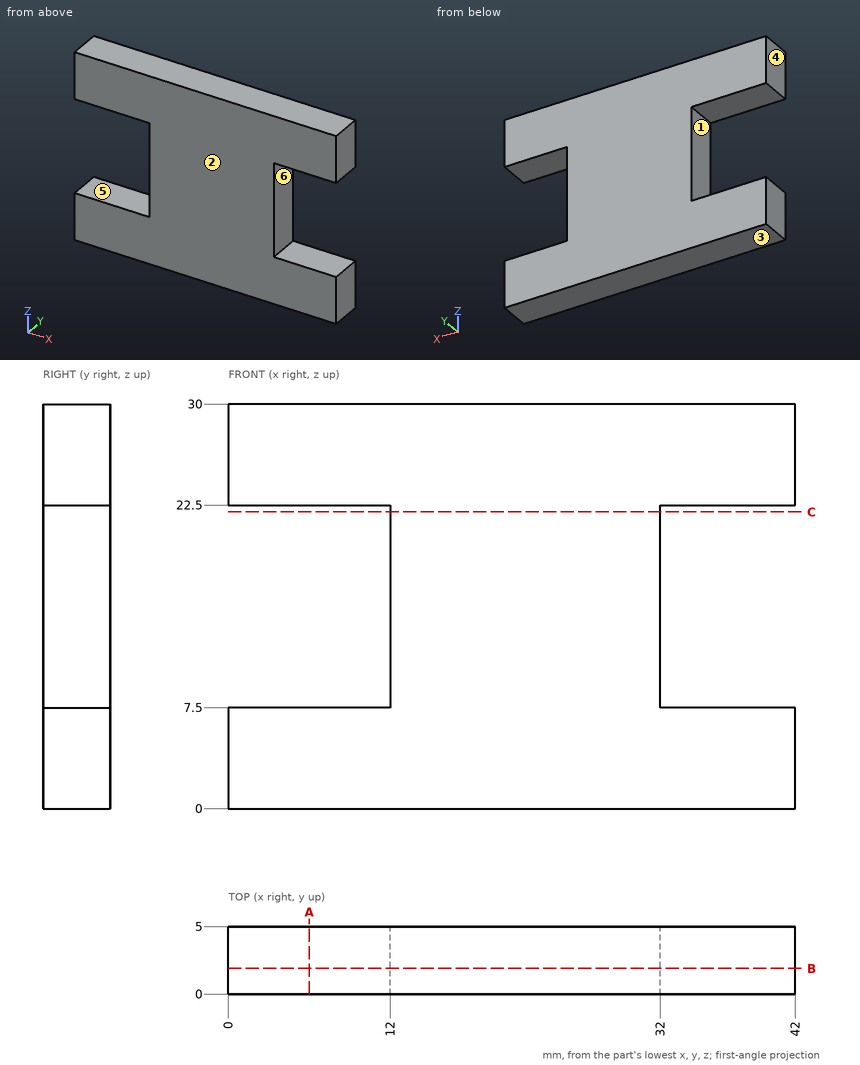
Part print with two shaded views. Sizes in mm from the minimum x, y, z corner. A direction names the side the tool comes from. Coordinates: 2 decimals unless noted, no trailing zeros. Write each loop counter-clockwise with the first axis right and the second up, starting at its lowest first coordinate (ties: lowest second). Pieces come first, ordered by that corner, then holes.
(1) Drill centre lines: line 1 (Z direction, x = 5, y = 4.2); line 2 (X direction, y = 2.25, z = 13.5). Where is each one in solid material? Low to high.
(2) Cut at A-A on x = 6. List the corners of the cut face in (y, z).
(3) 3-axis set-ups, long thin cutter, end or side, ignore diameter. For the marked faces 4, 5 and 6: which of +Z, -Z, +X, -X, +Y, -Y reach the whole face in a straight line?
(4) Mould opens along Z. For the marked faces 1, 2 and 3 say: pulls with the +Z half, pulls with the -Z half, needs draft (parallel to the pull), parting line crosses it, or undercut.
(5) Cut at C-C on z = 22. List the corners of the cut face in (x, y), and give its area (3 significant figures).
(6) Pin check, flat tip, straight feed: pin 1 Ø12 at (x, z) = (35.5, 13) entering from -Y. Stop position of the tip, or through.
(7) Cut at B-B on y = 1.9. List the corners of the cut face in (x, z).
Working result:
1. line 1: z = 0 to 7.5, 22.5 to 30
1. line 2: x = 12 to 32
2. outline: (0, 0) - (5, 0) - (5, 7.5) - (0, 7.5) - close; (0, 22.5) - (5, 22.5) - (5, 30) - (0, 30) - close
3. face 4: +Z, -Z, -X, +Y, -Y
3. face 5: -X, +Y, -Y
3. face 6: +X, +Y, -Y
4. face 1: undercut
4. face 2: needs draft
4. face 3: pulls with the -Z half
5. outline: (12, 0) - (32, 0) - (32, 5) - (12, 5) - close
5. area: 100 mm2
6. pin 1: stops at y = 0
7. outline: (0, 0) - (42, 0) - (42, 7.5) - (32, 7.5) - (32, 22.5) - (42, 22.5) - (42, 30) - (0, 30) - (0, 22.5) - (12, 22.5) - (12, 7.5) - (0, 7.5) - close
